```python
from build123d import *

# Parameters (mm, degrees)
SKETCH1_R           = 22.225
SKETCH1_R_2         = 15.875
BOSS_EXTRUDE1_DEPTH = 25.4
BOSS_EXTRUDE2_START = 2.54
SKETCH2_R           = 22.225
BOSS_EXTRUDE2_DEPTH = 2.54
BOSS_EXTRUDE3_START = 5.08
SKETCH3_R           = 15.875
BOSS_EXTRUDE3_DEPTH = 5.08
BOSS_EXTRUDE4_START = -13.208
SKETCH5_R           = 13.15140871
SKETCH5_R_2         = 11.43
BOSS_EXTRUDE4_DEPTH = 13.208


with BuildPart() as part:
    # Sketch1 → Boss-Extrude1 (new body)
    with BuildSketch(Plane(origin=(0, 0, 0), x_dir=(1, 0, 0), z_dir=(0, 1, 0))):
        with Locations(Location((0, 0, 0), (0, 0, 270))):
            Circle(SKETCH1_R)
        with Locations(Location((0, 0, 0), (0, 0, 270))):
            Circle(SKETCH1_R_2, mode=Mode.SUBTRACT)
    extrude(amount=BOSS_EXTRUDE1_DEPTH)

    # Sketch2 → Boss-Extrude2 (add)
    with BuildSketch(Plane.XZ.offset(BOSS_EXTRUDE2_START)):
        with Locations(Location((0, 0, 0), (0, 0, 270))):
            Circle(SKETCH2_R)
    extrude(amount=-BOSS_EXTRUDE2_DEPTH)

    # Sketch3 → Boss-Extrude3 (add)
    with BuildSketch(Plane.XZ.offset(2.54).offset(BOSS_EXTRUDE3_START)):
        with Locations(Location((0, 0, 0), (0, 0, 90))):
            Circle(SKETCH3_R)
    extrude(amount=-BOSS_EXTRUDE3_DEPTH)

    # Sketch4 → Revolve1 (revolve)
    with BuildSketch(Plane.XY):
        Polygon((-38.473670365, -51.398351826), (-9.898670365, -1.905), (-6.599113577, -3.81), (-35.174113577, -53.303351826), align=None)
    revolve1 = revolve(axis=Axis((0, -7.62, 0), (-0.500000000000001, -0.8660254037844382, 0)))

    # Sketch5 → Boss-Extrude4 (add)
    with BuildSketch(Plane(origin=(-31.874556788, -55.208351826, 0), x_dir=(0.866025403784438, -0.5000000000000012, 0), z_dir=(-0.5000000000000011, -0.8660254037844379, 0)).offset(BOSS_EXTRUDE4_START)):
        with Locations((3.81, 0)):
            Circle(SKETCH5_R)
        with Locations(Location((3.81, 0, 0), (0, 0, 90))):
            Circle(SKETCH5_R_2, mode=Mode.SUBTRACT)
    boss_extrude4 = extrude(amount=BOSS_EXTRUDE4_DEPTH)

    # Mirror1: Revolve1, Boss-Extrude4 across plane
    add(revolve1.mirror(Plane(origin=(0, 0, 0), x_dir=(0, 0, 1), z_dir=(1, 0, 0))))
    add(boss_extrude4.mirror(Plane(origin=(0, 0, 0), x_dir=(0, 0, 1), z_dir=(1, 0, 0))))


solid = part.part
```
Here's how the part is built. I have some questions about the finished solid (model axes, mm). A direction names the side the tool comes from. Coordinates: 2 decimals unless noted, no trailing zeros. Order: outer loops, then holes, each group sorted by start corner. A loop starts at its lowest first (then second) coordinate and runs counter-clockwise, first axis right, second up. Notation, with made-up numbers: (33.5, 75) - (85.5, 75) arc R9 cw to (85.5, 85) - close; hole circle Ø6 at (19, 28.5). An arc over 180 degrees is marked (long way). One line per question, with ' | ' between items. Start each with the question number.
1. If we mould it in two halves opening along Y, with no side actions, what happens to faces 4 (the cylindrical face through (36.605, -44.745, 0.578)), 5 (the cylindrical face through (-6.95, -18.44, -0.12)), 6 (the cylindrical face through (-23.758, -34.693, 2.919)), 7 (the flat face through (0, 0, 0))? For each: released by +Y, released by -Y, zero draft, split by the parting line, or undercut.
2. Please list where these lines run through material, in increasing order: line 1 along X through (y, z) = (6, 0) (3 decimals); line 2 along X through (y, z) = (-21.5, -2); line 3 along Y through (x, z) = (-6.5, 4.5). Write a range as [from, to].
3. If we section it at B-B (y = -21): Give the number of separate pieces and of enclosed holes in the cut face, and give its area (3 significant figures).
4. If we section it at C-C (z = -9.5): Write out the boundary of the cut face in (x, y).
5. I'm going to push flat-ended pins straight in: pin 1 Ø10 at (x, z) = (-31.5, -10.5) entering from +Y; pin 2 Ø9.5 at (x, z) = (2.5, -4) entering from -Y; pin 3 Ø5 at (y, z) = (9, -4) entering from +X. Where does each tip first touch, or does it pass through?
6. Which directions (+Z, -Z, +X, -X, +Y, -Y) give clear straight access to the entire face, cutting with the end or side of a thin tool? Please do faces 1 (the flat face through (-15, 25.4, 10)), 2 (the flat face through (-15, -2.54, -10)), 3 (the cylindrical face through (-15.497, 12.522, -3.441)).
7. If we section it at A-A (z = -14.5): Write out the boundary of the cut face in (x, y).
Model answer:
1) face 4: split by the parting line | face 5: undercut | face 6: undercut | face 7: released by +Y
2) line 1: x = [-22.225, -15.875], [15.875, 22.225] | line 2: x = [-21.01, -16.5], [-4.98, -0.48], [0.48, 4.98], [16.5, 21.01] | line 3: y = [-39.89, -31.18], [-17.38, -11.37], [-7.62, 0]
3) separate pieces: 1 | enclosed holes: 3 | area: 493 mm²
4) outline: (-36.45, -52.57) - (-20.7, -61.66) - (-14.09, -50.22) - (-16.47, -48.85) - (0, -20.33) - (16.47, -48.85) - (14.09, -50.22) - (20.7, -61.66) - (36.45, -52.57) - (29.85, -41.13) - (27.48, -42.5) - (7.34, -7.62) - (12.72, -7.62) - (12.72, -2.54) - (20.09, -2.54) - (20.09, 25.4) - (12.72, 25.4) - (12.72, 0) - (-12.72, 0) - (-12.72, 25.4) - (-20.09, 25.4) - (-20.09, -2.54) - (-12.72, -2.54) - (-12.72, -7.62) - (-7.34, -7.62) - (-27.48, -42.5) - (-29.85, -41.13) - close
5) pin 1: stops at y = -37.91 | pin 2: stops at y = -42.08 | pin 3: stops at x = 22.17
6) face 1: +Z, -Z, +X, -X, +Y | face 2: none | face 3: +Y
7) outline: (-16.84, -2.54) - (-6.46, -2.54) - (-6.46, -7.62) - (6.46, -7.62) - (6.46, -2.54) - (16.84, -2.54) - (16.84, 25.4) - (6.46, 25.4) - (6.46, 0) - (-6.46, 0) - (-6.46, 25.4) - (-16.84, 25.4) - close
